from build123d import *

# Parameters (mm, degrees)
BOSS_EXTRUDE1_DEPTH                              = 75
CBORE_FOR_M3_HEX_HEAD_MACHINE_SCREW2_D           = 3.5
CBORE_FOR_M3_HEX_HEAD_MACHINE_SCREW2_DEPTH       = 6.5
CBORE_FOR_M3_HEX_HEAD_MACHINE_SCREW2_CBORE_D     = 6
CBORE_FOR_M3_HEX_HEAD_MACHINE_SCREW2_CBORE_DEPTH = 3.5
LPATTERN2_COUNT                                  = 4
LPATTERN2_PITCH                                  = 20


with BuildPart() as part:
    # Sketch1 → Boss-Extrude1 (new body)
    with BuildSketch(Plane(origin=(67.5, 0, 0), x_dir=(0, 0, -1), z_dir=(1, 0, 0))):
        with BuildLine():
            Line((-3.441696476, -4.5), (-0.4, -4.5))
            Line((-0.4, -4.5), (0, -4.1))
            Line((0, -4.1), (0, 1.4))
            ThreePointArc((0, 1.4), (-0.2, 1.8), (0, 2.2))
            Line((0, 2.2), (0, 4.1))
            Line((0, 4.1), (-0.4, 4.5))
            Line((-0.4, 4.5), (-3.441696476, 4.5))
            ThreePointArc((-3.441696476, 4.5), (-3.524448068, 4.475108648), (-3.579735674, 4.408695652))
            ThreePointArc((-3.579735674, 4.408695652), (-3.747623907, 4.141262777), (-3.990528855, 3.939510483))
            ThreePointArc((-3.990528855, 3.939510483), (-4.041057421, 3.890337026), (-4.063537838, 3.823510417))
            Line((-4.063537838, 3.823510417), (-4.09336636, 3.482568852))
            ThreePointArc((-4.09336636, 3.482568852), (-4.157487258, 3.352544533), (-4.292605299, 3.3))
            Line((-4.292605299, 3.3), (-4.707394701, 3.3))
            ThreePointArc((-4.707394701, 3.3), (-4.842512742, 3.352544533), (-4.90663364, 3.482568852))
            Line((-4.90663364, 3.482568852), (-4.93646249, 3.823514163))
            ThreePointArc((-4.93646249, 3.823514163), (-4.958942652, 3.890340367), (-5.009470648, 3.939513741))
            ThreePointArc((-5.009470648, 3.939513741), (-5.252372199, 4.141265182), (-5.420258326, 4.408695652))
            ThreePointArc((-5.420258326, 4.408695652), (-5.475545932, 4.475108648), (-5.558297524, 4.5))
            Line((-5.558297524, 4.5), (-6.1, 4.5))
            Line((-6.1, 4.5), (-6.5, 4.1))
            Line((-6.5, 4.1), (-6.5, -4.1))
            Line((-6.5, -4.1), (-6.1, -4.5))
            Line((-6.1, -4.5), (-5.558297524, -4.5))
            ThreePointArc((-5.558297524, -4.5), (-5.475545932, -4.475108648), (-5.420258326, -4.408695652))
            ThreePointArc((-5.420258326, -4.408695652), (-5.252372199, -4.141265182), (-5.009470648, -3.939513741))
            ThreePointArc((-5.009470648, -3.939513741), (-4.958942652, -3.890340367), (-4.93646249, -3.823514163))
            Line((-4.93646249, -3.823514163), (-4.90663364, -3.482568852))
            ThreePointArc((-4.90663364, -3.482568852), (-4.842512742, -3.352544533), (-4.707394701, -3.3))
            Line((-4.707394701, -3.3), (-4.292605299, -3.3))
            ThreePointArc((-4.292605299, -3.3), (-4.157487258, -3.352544533), (-4.09336636, -3.482568852))
            Line((-4.09336636, -3.482568852), (-4.063537838, -3.823510417))
            ThreePointArc((-4.063537838, -3.823510417), (-4.041057421, -3.890337026), (-3.990528855, -3.939510483))
            ThreePointArc((-3.990528855, -3.939510483), (-3.747623907, -4.141262777), (-3.579735674, -4.408695652))
            ThreePointArc((-3.579735674, -4.408695652), (-3.524448068, -4.475108648), (-3.441696476, -4.5))
        make_face()
    extrude(amount=-BOSS_EXTRUDE1_DEPTH)

    # CBORE for M3 Hex Head Machine Screw2
    with Locations(Plane.XY.offset(6.5)):
        with Locations((0, 0)):
            cbore_for_m3_hex_head_machine_screw2 = CounterBoreHole(CBORE_FOR_M3_HEX_HEAD_MACHINE_SCREW2_D / 2, CBORE_FOR_M3_HEX_HEAD_MACHINE_SCREW2_CBORE_D / 2, CBORE_FOR_M3_HEX_HEAD_MACHINE_SCREW2_CBORE_DEPTH, depth=CBORE_FOR_M3_HEX_HEAD_MACHINE_SCREW2_DEPTH)

    # LPattern2: CBORE for M3 Hex Head Machine Screw2 ×4
    with Locations(*[(i * LPATTERN2_PITCH, 0, 0) for i in range(1, LPATTERN2_COUNT)]):
        add(cbore_for_m3_hex_head_machine_screw2, mode=Mode.SUBTRACT)


solid = part.part
Part model, mm, in its own coordinate system. A direction names the side the tool comes from. Give positions to 0.01 mm unless a question says otherwise; leave off trailing zeros. Write each question's results on one line, items separated by ' | '. Start each with the question number.
Q1. Pull direction X, two halves, no side cores. Call faces 1 (the face through (59.19, -1.55, 1.48)), 2 (the face through (67.5, 0, 3)), 3 (the face through (31, 0, 6.5)): +X half, -X half, draft (parallel to the pull), parting line (faces both ways), or undercut.
Q2. Which spindle directions (+Z, -Z, +X, -X, +Y, -Y) get a long thin tool onto all of the face, cutting with end or side? Do faces 4 (the face through (39.19, -1.55, 1.48)), 5 (the face through (42, 0, 3)). Say none if no direction does.
Q3. Pin check, flat tips, straight feed: P1, Ø3, axis at x = 40, y = 0, coming from the +Z side; P2, Ø4, axis at x = 0, y = 0, coming from the +Z side. Stop position of each tip, or through.
Q4. Band-saw the part on B-B on y = 0. Count the separate pieces of the cut face and the enclosed holes in it, plus the area to 4 significant figures.
Q5. Wall check: L1, parallel to X at y = -0.25, z = 5.5; L2, parallel to Y at x = 60, z = 1.6; L3, parallel to X at y = 0, z = 1. Give the ranges that are in metal, low to high.
Results are:
1) face 1: undercut | face 2: +X half | face 3: draft
2) face 4: +Z, -Z | face 5: +Z
3) P1: passes through | P2: stops at z = 3
4) separate pieces: 5 | enclosed holes: 0 | area: 361.5 mm²
5) L1: x = -7.5 to -2.99, 2.99 to 17.01, 22.99 to 37.01, 42.99 to 57.01, 62.99 to 67.5 | L2: y = -4.5 to -1.75, 1.75 to 4.5 | L3: x = -7.5 to -1.75, 1.75 to 18.25, 21.75 to 38.25, 41.75 to 58.25, 61.75 to 67.5
